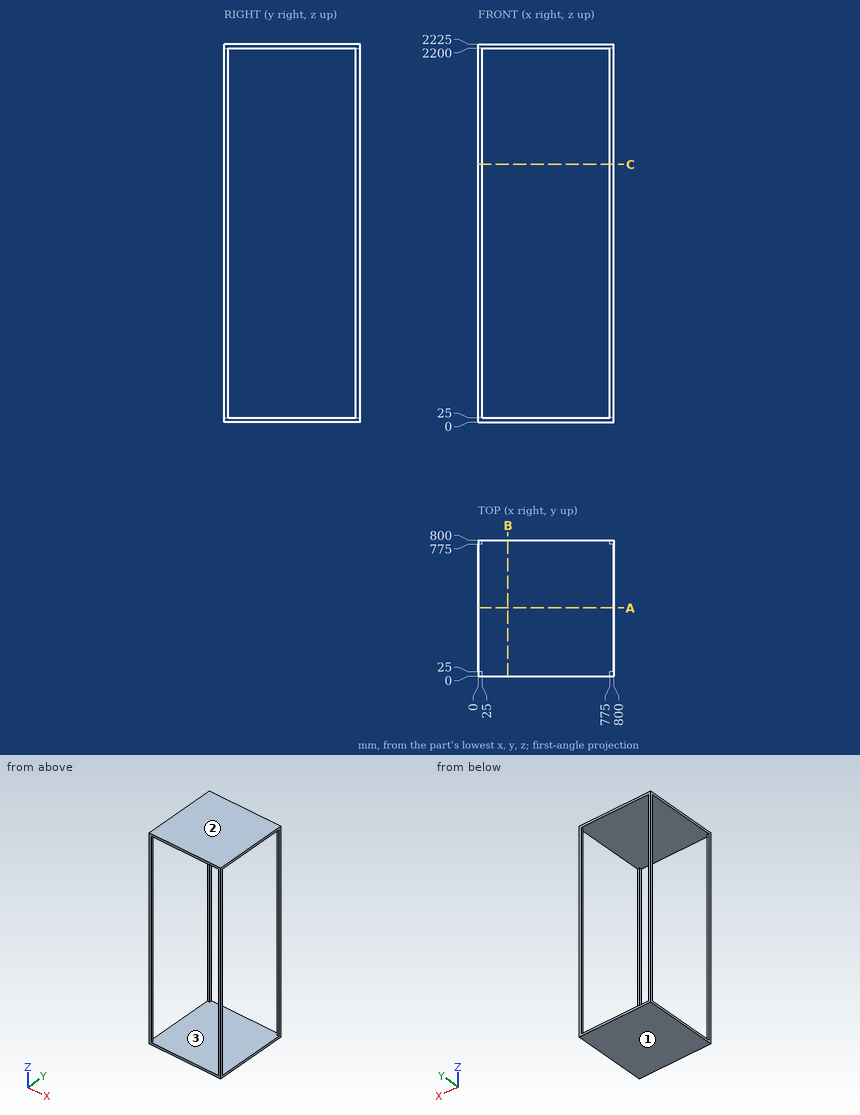
Could you check a few things on this drawing? It's one solid part, dimensions in mm from its lowest x, y, z. Round coordinates to 2 decimals unless told otherwise and drop trailing zeros. Order: outer loops, then holes, each group sorted by start corner. A loop starts at its lowest first (then second) coordinate and runs counter-clockwise, first axis right, second up. Notation, with made-up numbers: M 26,-23 L 46,-23 A10 ccw 46,-11 Z; hole C 3,37.5 d5. An arc over 180 degrees is marked long. One line per item, written item: value.
(1) If we mould it in two halves opening along Z, with no side actions, what happens to the marked faces 1, 2 and 3? For each: released by +Z, released by -Z, zero draft, split by the parting line, or undercut.
Ans:
face 1: released by -Z
face 2: released by +Z
face 3: undercut
(2) Imagine slicing it at C-C (z = 1516.5). Write out the boundary of the cut face in (x, y).
Ans:
outline: M 0,0 L 25,0 L 25,25 L 0,25 Z; M 0,775 L 25,775 L 25,800 L 0,800 Z; M 775,0 L 800,0 L 800,25 L 775,25 Z; M 775,775 L 800,775 L 800,800 L 775,800 Z
(3) Imagine slicing it at A-A (y = 400.5). Write out the boundary of the cut face in (x, z).
Ans:
outline: M 0,0 L 800,0 L 800,25 L 0,25 Z; M 0,2200 L 800,2200 L 800,2225 L 0,2225 Z
(4) I need wall thicknesses on line 1 along Z through (x, y) = (43, 373). Which ranges of the line are inside material? Lowest first, please. Write a range as from..to.
Ans:
line 1: z = 0..25, 2200..2225
